Read the model definition and answer for the solid it produces. Units are mm, in the model's axes. Give positions to 0.01 mm unless a question says otherwise; leave off trailing zeros. Order: outer loops, then holes, each group sorted by start corner. A loop starts at its lowest first (then second) coordinate and runs counter-clockwise, first axis right, second up. Notation, with made-up numbers: M -11.5,-24.75 L 31.5,-24.75 A22 ccw 31.5,-8.75 Z; hole C -34.5,-11 d4. An arc over 180 degrees is marked long. One line per item, written item: value.
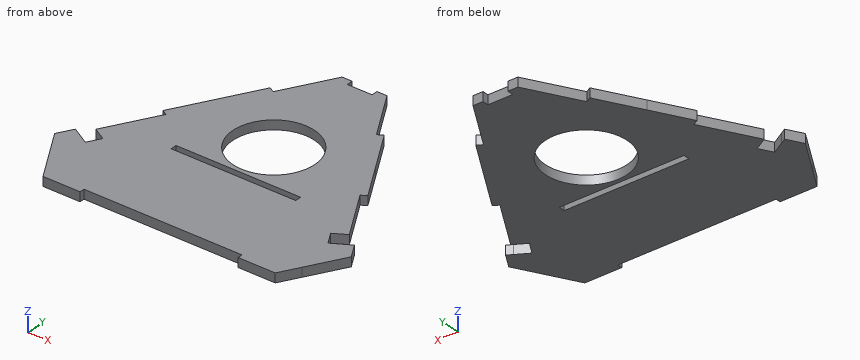
from build123d import *

# Parameters (mm, degrees)
BOSS_EXTRUDE1_DEPTH     = 4.7625
SCALE2_SCALE_X          = 0.25
SCALE2_SCALE_Y          = 0.25
SCALE2_SCALE_Z          = 1
SKETCH8_R               = 21.082
CUT_EXTRUDE5_DEPTH      = 286.136245759
CUT_EXTRUDE8_DEPTH      = 286.136245759
CUT_EXTRUDE8_DEPTH_BACK = 286.136245759
SKETCH9_W               = 64.0334
SKETCH9_H               = 3.2004
SKETCH10_W              = 12.7
SKETCH10_H              = 3.175
CUT_EXTRUDE9_DEPTH      = 286.136245759
CUT_EXTRUDE10_DEPTH     = 286.136245759
CUT_EXTRUDE11_DEPTH     = 286.136245759
CUT_EXTRUDE12_DEPTH     = 286.136245759
SKETCH18_W              = 40.580539391
SKETCH18_H              = 7.62
BOSS_EXTRUDE2_DEPTH     = 4.7625
CUT_EXTRUDE13_REACH     = 286.64


with BuildPart() as part:
    # Sketch3 → Boss-Extrude1 (new body)
    with BuildSketch(Plane.XY):
        Polygon((312.000738686, 65.991135768), (166.792028218, 317.5), (-166.792028218, 317.5), (-312.000738686, 65.991135768), (-276.650369343, 4.7625), (276.650369343, 4.7625), align=None)
        Polygon((-166.792028218, 317.5), (166.792028218, 317.5), (60.750369343, 501.169540891), (-60.750369343, 501.169540891), align=None)
    extrude(amount=BOSS_EXTRUDE1_DEPTH)


with BuildPart() as part_1:
    # Scale2: scaled about (0, 198.568597006, 2.38125)
    add(part.part.scale((SCALE2_SCALE_X, SCALE2_SCALE_Y, SCALE2_SCALE_Z), about=(0, 198.568597006, 2.38125)))

    # Sketch8 → Cut-Extrude5 (cut, through all)
    with BuildSketch(Plane.XY.offset(4.7625)):
        with Locations((0, 214.887072754)):
            Circle(SKETCH8_R)
    extrude(amount=-CUT_EXTRUDE5_DEPTH, mode=Mode.SUBTRACT)

    # Sketch9 → Cut-Extrude8 (cut, two sides: drawn at the far end of the back side and taken through both)
    with BuildSketch(Plane.XY.offset(4.7625).offset(-CUT_EXTRUDE8_DEPTH_BACK)):
        with Locations((0, 190.118897754)):
            Rectangle(SKETCH9_W, SKETCH9_H)
    extrude(amount=CUT_EXTRUDE8_DEPTH + CUT_EXTRUDE8_DEPTH_BACK, mode=Mode.SUBTRACT)

    # Sketch10 → Cut-Extrude9 (cut, through all)
    with BuildSketch(Plane.XY.offset(4.7625)):
        with Locations((0, 272.631332977)):
            Rectangle(SKETCH10_W, SKETCH10_H)
    extrude(amount=-CUT_EXTRUDE9_DEPTH, mode=Mode.SUBTRACT)

    # Sketch11 → Cut-Extrude10 (cut, through all)
    with BuildSketch(Plane.XY.offset(4.7625)):
        Polygon((15.187592336, 274.218832977), (29.284592336, 249.802112743), (26.534961679, 248.214612743), (11.521418126, 274.218832977), align=None)
        Polygon((-29.284592336, 249.802112743), (-26.534961679, 248.214612743), (-11.521418126, 274.218832977), (-15.187592336, 274.218832977), align=None)
    extrude(amount=-CUT_EXTRUDE10_DEPTH, mode=Mode.SUBTRACT)

    # Sketch12 → Cut-Extrude11 (cut, through all)
    with BuildSketch(Plane.XY.offset(4.7625)):
        Polygon((71.650184671, 176.422754325), (52.600184671, 209.418322209), (49.850554014, 207.830822209), (68.900554014, 174.835254325), align=None)
        Polygon((-71.650184671, 176.422754325), (-68.900554014, 174.835254325), (-49.850554014, 207.830822209), (-52.600184671, 209.418322209), align=None)
    extrude(amount=-CUT_EXTRUDE11_DEPTH, mode=Mode.SUBTRACT)

    # Sketch13 → Cut-Extrude12 (cut, through all)
    with BuildSketch(Plane.XY.offset(4.7625)):
        Polygon((78.000184671, 165.424231696), (76.167097567, 168.599231696), (62.550554014, 145.01468644), (65.300184671, 143.42718644), align=None)
        Polygon((-62.550554014, 145.01468644), (-65.300184671, 143.42718644), (-78.000184671, 165.424231696), (-76.167097567, 168.599231696), align=None)
    extrude(amount=-CUT_EXTRUDE12_DEPTH, mode=Mode.SUBTRACT)

    # Sketch18 → Boss-Extrude2 (add)
    with BuildSketch(Plane(origin=(0, 0, 0), x_dir=(-1, 0, 0), z_dir=(0, 0, -1))):
        Polygon((-40.580539391, 150.117072754), (-65.496418126, 150.117072754), (-59.630539391, 139.957072754), (-40.580539391, 139.957072754), (-40.580539391, 142.497072754), align=None)
        with Locations((-20.290269696, 146.307072754)):
            Rectangle(SKETCH18_W, SKETCH18_H)
        with Locations((20.290269696, 146.307072754)):
            Rectangle(SKETCH18_W, SKETCH18_H)
        Polygon((65.496418126, 150.117072754), (40.580539391, 150.117072754), (40.580539391, 142.497072754), (40.580539391, 139.957072754), (59.630539391, 139.957072754), align=None)
    extrude(amount=-BOSS_EXTRUDE2_DEPTH)

    # Sketch20 → Cut-Extrude13 (cut, up to next)
    with BuildSketch(Plane(origin=(0, 0, 0), x_dir=(-1, 0, 0), z_dir=(0, 0, -1)), mode=Mode.PRIVATE) as cut_extrude13_sk1:
        Polygon((68.900554014, 174.835254325), (65.090554014, 181.434367901), (58.491440438, 177.624367901), (62.301440438, 171.025254325), align=None)
    cut_extrude13_tool1 = extrude(cut_extrude13_sk1.sketch, amount=-CUT_EXTRUDE13_REACH, mode=Mode.PRIVATE) & part_1.part
    cut_extrude13 = cut_extrude13_tool1.solids().sort_by_distance((-63.695997, 176.229811, 0))[0]
    add(cut_extrude13, mode=Mode.SUBTRACT)

    # Mirror1: Cut-Extrude13 across plane
    add(cut_extrude13.mirror(Plane(origin=(0, 0, 0), x_dir=(0, 0, 1), z_dir=(1, 0, 0))), mode=Mode.SUBTRACT)


solid = part_1.part
1) Find section B-B, the plane y = 205. Write down the section's boundary in (x, z), plus the area to 3 significant figures.
Reported:
outline: M -51.48,0 L -18.62,0 L -18.62,4.76 L -51.48,4.76 Z; M 18.62,0 L 51.48,0 L 51.48,4.76 L 18.62,4.76 Z
area: 313 mm^2
2) Find section C-C, the plane x = -16.5. Write down the section's boundary in (y, z).
Reported:
outline: M 142.5,0 L 188.52,0 L 188.52,4.76 L 142.5,4.76 Z; M 191.72,0 L 201.76,0 L 201.76,4.76 L 191.72,4.76 Z; M 228.01,0 L 265.6,0 L 265.6,4.76 L 228.01,4.76 Z
3) Find section D-D, the plane z = 3.95. Count the separate pieces of the cut face and the enclosed holes in it, plus the area to 3 significant figures.
Reported:
separate pieces: 1
enclosed holes: 2
area: 11,100 mm^2
4) Find section A-A, the plane x = 0. Write down the section's boundary in (y, z).
Reported:
outline: M 142.5,0 L 188.52,0 L 188.52,4.76 L 142.5,4.76 Z; M 191.72,0 L 193.81,0 L 193.81,4.76 L 191.72,4.76 Z; M 235.97,0 L 271.04,0 L 271.04,4.76 L 235.97,4.76 Z
5) Consider probe 1 along Y at (x, z) = (0, 3.15); probe 2 along Y at (x, z) = (-9.5, 1.9); probe 3 along X at (y, z) = (221.5, 4.05). Determine where each line is inside the solid, lowest interval first.
Reported:
probe 1: y = 142.5 to 188.52, 191.72 to 193.81, 235.97 to 271.04
probe 2: y = 142.5 to 188.52, 191.72 to 196.07, 233.71 to 274.22
probe 3: x = -45.62 to -20.02, 20.02 to 45.62
6) Each of these flat-tipped pins is pushed along its axis until it touches: pin 1 Ø1.6 at (y, z) = (273, 3) entering from -X; pin 2 Ø1.4 at (x, z) = (10.5, 3) entering from -Y; pin 3 Ø2 at (y, z) = (238.5, 2.5) entering from +X. Where does it stop, or does it pass through?
Reported:
pin 1: stops at x = -12.69
pin 2: stops at y = 142.5
pin 3: stops at x = 36.39
